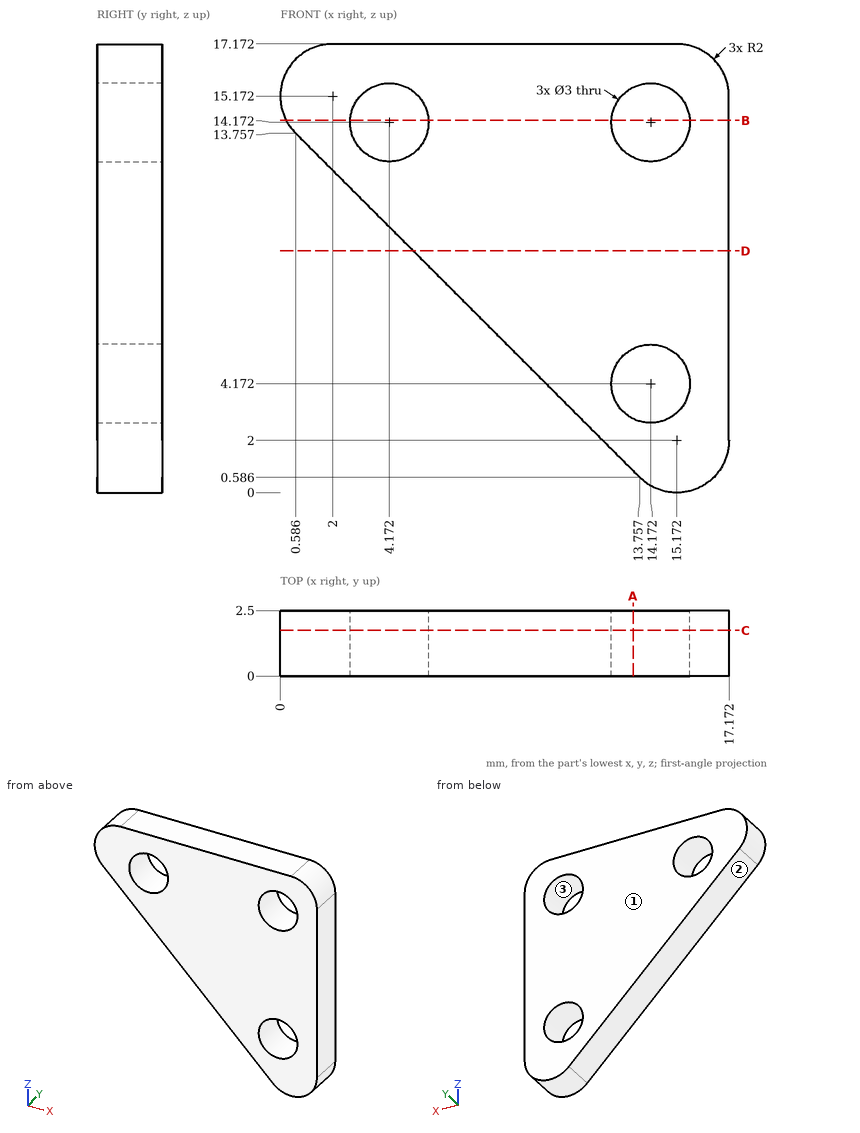
Answer from the drawing. Dimensions are ordinates in mm from the lowest x, y and z of the part. Round coordinates to 2 decimals unless told otherwise and drop trailing zeros. Write each loop counter-clockwise with the first axis right and the second up, starting at its lowest first coordinate (ties: lowest second). Pieces come first, ordered by that corner, then holes. Notation, with made-up numbers: (-23, 8.5) -> (-19, 8.5) arc R22 cw to (-19, 43.5) -> close; hole circle Ø3 at (71.5, 4.25). An arc over 180 degrees is marked (long way). Answer in a Markdown table with one row per item. Add a question column.
1) Find section A-A, the plane x = 13.5. Determine the outline of the cut face in (y, z).
2) Find section C-C, the plane y = 1.75. Determine the outline of the cut face in (x, z) (1 decimal).
3) Find section B-B, the plane z = 14.25. Determine the outline of the cut face in (x, y) (1 decimal), and give its area (3 significant figures).
4) Find section D-D, the plane z = 9.25. Determine the outline of the cut face in (x, y), and give its area (3 significant figures).
5) Consider line 1 (X direction, y = 1.1, z = 13.5) (1 decimal); line 2 (X direction, y = 1.35, z = 15.25) (1 decimal); line 3 (Z direction, x = 13, y = 0.5) (1 decimal). Determine where each line is inside the solid, lowest interval first.
6) Determine the mould class of the marked faces 1, 2 and 3 for opening direction X: pulls with the +X half, pulls with the -X half, needs draft (parallel to the pull), parting line crosses it, or undercut.
Findings below:
| question | item | result |
|---|---|---|
| 1 | outline | (0, 0.84) -> (2.5, 0.84) -> (2.5, 2.83) -> (0, 2.83) -> close; (0, 5.51) -> (2.5, 5.51) -> (2.5, 12.83) -> (0, 12.83) -> close; (0, 15.51) -> (2.5, 15.51) -> (2.5, 17.17) -> (0, 17.17) -> close |
| 2 | outline | (0.6, 13.8) -> (13.8, 0.6) arc R2 ccw to (17.2, 2) -> (17.2, 15.2) arc R2 ccw to (15.2, 17.2) -> (2, 17.2) arc R2 ccw to start; hole circle Ø3 at (4.2, 14.2); hole circle Ø3 at (14.2, 4.2); hole circle Ø3 at (14.2, 14.2) |
| 3 | outline | (0.2, 0) -> (2.7, 0) -> (2.7, 2.5) -> (0.2, 2.5) -> close; (5.7, 0) -> (12.7, 0) -> (12.7, 2.5) -> (5.7, 2.5) -> close; (15.7, 0) -> (17.2, 0) -> (17.2, 2.5) -> (15.7, 2.5) -> close |
| 3 | area | 27.4 mm² |
| 4 | outline | (5.09, 0) -> (17.17, 0) -> (17.17, 2.5) -> (5.09, 2.5) -> close |
| 4 | area | 30.2 mm² |
| 5 | line 1 | 0.8 to 2.8, 5.5 to 12.8, 15.5 to 17.2 |
| 5 | line 2 | 0 to 3.1, 5.2 to 13.1, 15.2 to 17.2 |
| 5 | line 3 | 1.3 to 3.2, 5.1 to 13.2, 15.1 to 17.2 |
| 6 | face 1 | needs draft |
| 6 | face 2 | pulls with the -X half |
| 6 | face 3 | undercut |
